```python
from build123d import *

# Parameters (mm, degrees)
SKETCH2_R                 = 12.7
SKETCH2_R_2               = 6
BOSS_EXTRUDE1_DEPTH       = 11
SKETCH3_R                 = 16
SKETCH3_R_2               = 6
BOSS_EXTRUDE2_DEPTH       = 3.175
M3X0_5_TAPPED_HOLE1_D     = 2.5
M3X0_5_TAPPED_HOLE1_DEPTH = 15
M3X0_5_TAPPED_HOLE1_TIP   = 0.751075774


with BuildPart() as part:
    # Sketch2 → Boss-Extrude1 (new body, symmetric)
    with BuildSketch(Plane.XY):
        Circle(SKETCH2_R)
        Circle(SKETCH2_R_2, mode=Mode.SUBTRACT)
    extrude(amount=BOSS_EXTRUDE1_DEPTH, both=True)

    # Sketch3 → Boss-Extrude2 (add)
    with BuildSketch(Plane(origin=(0, 0, -11), x_dir=(-1, 0, 0), z_dir=(0, 0, -1))):
        Circle(SKETCH3_R)
        Circle(SKETCH3_R_2, mode=Mode.SUBTRACT)
    extrude(amount=BOSS_EXTRUDE2_DEPTH)

    # M3x0.5 Tapped Hole1
    with Locations(Plane.XY.offset(11)):
        with Locations((-8, 5), (-8, -5), (8, -5), (8, 5)):
            Hole(M3X0_5_TAPPED_HOLE1_D / 2, depth=M3X0_5_TAPPED_HOLE1_DEPTH)
            with Locations((0, 0, -(M3X0_5_TAPPED_HOLE1_DEPTH + M3X0_5_TAPPED_HOLE1_TIP / 2))):  # 118° drill point
                Cone(0, M3X0_5_TAPPED_HOLE1_D / 2, M3X0_5_TAPPED_HOLE1_TIP, mode=Mode.SUBTRACT)


solid = part.part
```
The listing builds one solid part. Answer for the finished solid, in the listing's coordinates (mm). A direction names the side the tool comes from. Coordinates: 2 decimals unless noted, no trailing zeros. Write each loop counter-clockwise with the first axis right and the second up, starting at its lowest first coordinate (ties: lowest second). Pieces come first, ordered by that corner, then holes. Notation, with made-up numbers: (-17.75, 77.5) - (41.25, 77.5) arc R27 cw to (41.25, 108.5) - close; hole circle Ø4 at (11.25, -8.75). An arc over 180 degrees is marked (long way). Return JSON: item names as keys, results as strings. Group by question number.
1. Determine the mould class of faces 1 (the conical face through (7.84, 5.15, -4.62)), 2 (the cylindrical face through (-2.75, -12.4, 0.15)), 3 (the flat face through (-7, 0, -14.175)) for opening direction Y: released by +Y, released by -Y, zero draft, split by the parting line, or undercut.
2. A cutting plane is placed at D-D, the plane y = -7.5. Determine the outline of the cut face in (x, z) (3 decimals), plus the area to 3 significant figures.
3. A cutting plane is placed at A-A, the plane x = 0. Determine the outline of the cut face in (y, z) (3 decimals).
4. A cutting plane is placed at C-C, the plane z = 0.25. Determine the outline of the cut face in (x, y), plus the area to 3 significant figures.
5. Straight lines are drawn through the part: L1, parallel to X at y = -5, z = 0; L2, parallel to Y at x = -8, z = 5.25; L3, parallel to Y at x = 0, z = -5.5. For each, find the intervals that lie inside material, in ascending order.
6. Given pin 1 (4 mm diameter, centred on x = -8, z = 5, fed in from +Y); pin 2 (1 mm diameter, centred on x = -9.5, z = 1.5, fed in from +Y); pin 3 (10 mm diameter, centred on x = 2.5, z = 7, fed in from +Y); pin 4 (11 mm diameter, centred on x = 0, y = 0, fed in from +Z), each flat-ended and moving along its own axis, determine where each tip first touches the part or whether it passes through.
7. Which of the six approach directions +Z, -Z, +X, -X, +Y, -Y give full straight-line access (tool end or side, diameter ignored) to faces 4 (the cylindrical face through (3.47, -15.62, -12.57)), 5 (the cylindrical face through (-7.01, -5.76, 3.39))?
Ans:
{
 "1": {"face 1": "undercut", "face 2": "split by the parting line", "face 3": "zero draft"},
 "2": {"outline": "(-14.133, -14.175) - (14.133, -14.175) - (14.133, -11) - (10.249, -11) - (10.249, 11) - (-10.249, 11) - (-10.249, -11) - (-14.133, -11) - close", "area": "541 mm²"},
 "3": {"outline": "(-16, -14.175) - (-6, -14.175) - (-6, 11) - (-12.7, 11) - (-12.7, -11) - (-16, -11) - close; (6, -14.175) - (16, -14.175) - (16, -11) - (12.7, -11) - (12.7, 11) - (6, 11) - close"},
 "4": {"outline": "circle Ø25.4 at (0, 0); hole circle Ø2.5 at (-8, -5); hole circle Ø2.5 at (-8, 5); hole circle Ø12 at (0, 0); hole circle Ø2.5 at (8, -5); hole circle Ø2.5 at (8, 5)", "area": "374 mm²"},
 "5": {"L1": "-11.67 to -9.25, -6.75 to -3.32, 3.32 to 6.75, 9.25 to 11.67", "L2": "-9.86 to -6.25, -3.75 to 3.75, 6.25 to 9.86", "L3": "-12.7 to -6, 6 to 12.7"},
 "6": {"pin 1": "y = 11.19", "pin 2": "y = 8.96", "pin 3": "y = 12.7", "pin 4": "through"},
 "7": {"face 4": "+Z, -Z", "face 5": "+Z"}
}
